Autodesk Inventor part; units mm, degrees
ref_plane "РабПлоскость1" through (0, 0, 6) normal (0, 0, 1) x (1, 0, 0)
ref_plane "YZ Plane" through (0, 0, 0) normal (1, 0, 0) x (0, 1, 0)
ref_plane "XZ Plane" through (0, 0, 0) normal (0, 1, 0) x (-1, 0, 0)
sketch "Эскиз1" plane through (0, 0, 0) normal (0, 0, 1) x (1, 0, 0)
  circle A0 centre (0, 0) radius 4
  line L0 (10.9362, 0) -> (5.4681, 9.471)
  line L1 (-5.4681, 9.471) -> (5.4681, 9.471)
  line L2 (-10.9362, 0) -> (-5.4681, 9.471)
  line L3 (-5.4681, -9.471) -> (5.4681, -9.471)
  line L4 (-5.4681, -9.471) -> (-10.9362, 0)
  line L5 (10.9362, 0) -> (5.4681, -9.471)
  line L6 (0, 0) -> (10.9362, 0)
  dimension "d45" = 8
  dimension "d52" = 120
  dimension "d53" = 120
  dimension "d54" = 10.9362
  dimension "d55" = 9.471
extrude "Выдавливание1" add sketch "Эскиз1" along normal blind 12
sketch "Эскиз3" plane through (0, 0, 12) normal (0, 0, 1) x (1, 0, 0)
  circle A0 centre (0, 0) radius 4
  circle A1 centre (0, 0) radius 5.5
  dimension "d56" = 8
  dimension "d57" = 11
extrude "Выдавливание3" add sketch "Эскиз3" along normal blind 1.5
chamfer "Фаска2" distance 0.5 angle 45 1 edges at (-5.5, 0, 13.5)
ref_plane "РабПлоскость1" through (0, 0, 6) normal (0, 0, 1) x (1, 0, 0)
mirror "Зеркальное отражение1" about plane through (0, 0, 6) normal (0, 0, 1) of "Выдавливание3"
chamfer "Фаска3" distance 0.5 angle 45 1 edges at (-5.5, 0, -1.5)
thread "Резьба1"
properties part number "Нагаечник"
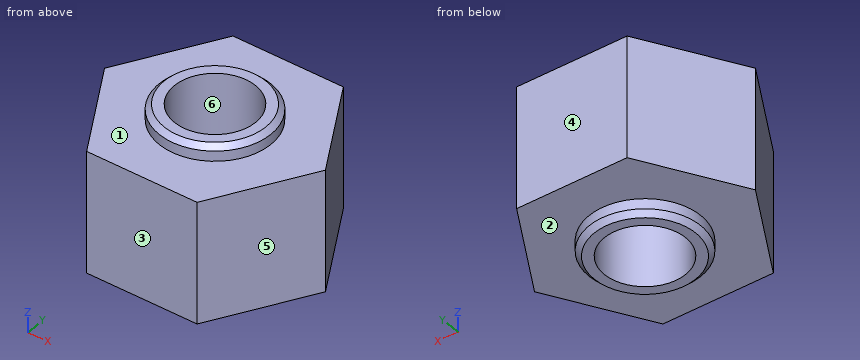
For this review, take the finished solid that the model builds, in its own axes (mm). Face numbers are marked on the shaded views. A direction names the side the tool comes from. Coordinates: 2 decimals unless noted, no trailing zeros. Write each loop counter-clockwise with the first axis right and the second up, starting at its lowest first coordinate (ties: lowest second). Pieces come first, ordered by that corner, then holes. Notation, with made-up numbers: (89, 53.25) -> (121, 53.25) arc R33 cw to (121, 89.25) -> close; hole circle Ø8 at (7.5, -24.5). An arc over 180 degrees is marked (long way). Write each question's results on one line, items separated by ' | '. Start each with the question number.
1) For the marked faces 1, 2 and 3, list the 3-axis set-ups (+Z, -Z, +X, -X, +Y, -Y) from which the entire face can be reached by the end or side of a thin tool; tool diameter is ignored.
2) Consider section A-A (x = 0). Write out the cut boundary in (y, z), plus the area to 3 significant figures.
3) The part is to be moulded in two halves that separate along X. For the marked faces 4, 5 and 6, say which applies: +X half, -X half, draft (parallel to the pull), parting line (faces both ways), or undercut.
4) Insertion check: pin 1 (3 mm diameter, centred on y = -4, z = 3, fed in from -X); pin 2 (2 mm diameter, centred on x = 7, z = 9, fed in from +Y); pin 3 (2 mm diameter, centred on y = 5.5, z = 1.5, fed in from -X). Each pin has a flat end and moves straight along its axis. Give the tip position at first contact, or say it passes through.
5) Wall thickness on L1, parallel to Y at x = 0, z = 5.75; L2, parallel to Z at x = 5.5, y = -1.25; L3, parallel to Y at x = -3.25, z = 3.5: over which ranges is each line inside the solid? List them lowest first. Write a range as [from, to].
6) Consider section C-C (y = -7). Write out the cut boundary in (x, z).
7) Consider section D-D (x = 6.5). Write out the cut boundary in (y, z).
8) Consider section B-B (z = 10.5). Write out the cut boundary in (x, y).
Geometry says:
1) face 1: +Z | face 2: -Z | face 3: +Z, -Z, +X, -X, -Y
2) outline: (-9.47, 0) -> (-5.5, 0) -> (-5.5, -1) -> (-5, -1.5) -> (-4, -1.5) -> (-4, 13.5) -> (-5, 13.5) -> (-5.5, 13) -> (-5.5, 12) -> (-9.47, 12) -> close; (4, -1.5) -> (5, -1.5) -> (5.5, -1) -> (5.5, 0) -> (9.47, 0) -> (9.47, 12) -> (5.5, 12) -> (5.5, 13) -> (5, 13.5) -> (4, 13.5) -> close | area: 140 mm^2
3) face 4: draft | face 5: +X half | face 6: undercut
4) pin 1: x = -9.49 | pin 2: y = 8.55 | pin 3: x = -8.34
5) L1: [-9.47, -4], [4, 9.47] | L2: [0, 12] | L3: [-9.47, -2.33], [2.33, 9.47]
6) outline: (-6.89, 0) -> (6.89, 0) -> (6.89, 12) -> (-6.89, 12) -> close
7) outline: (-7.68, 0) -> (7.68, 0) -> (7.68, 12) -> (-7.68, 12) -> close
8) outline: (-10.94, 0) -> (-5.47, -9.47) -> (5.47, -9.47) -> (10.94, 0) -> (5.47, 9.47) -> (-5.47, 9.47) -> close; hole circle Ø8 at (0, 0)
